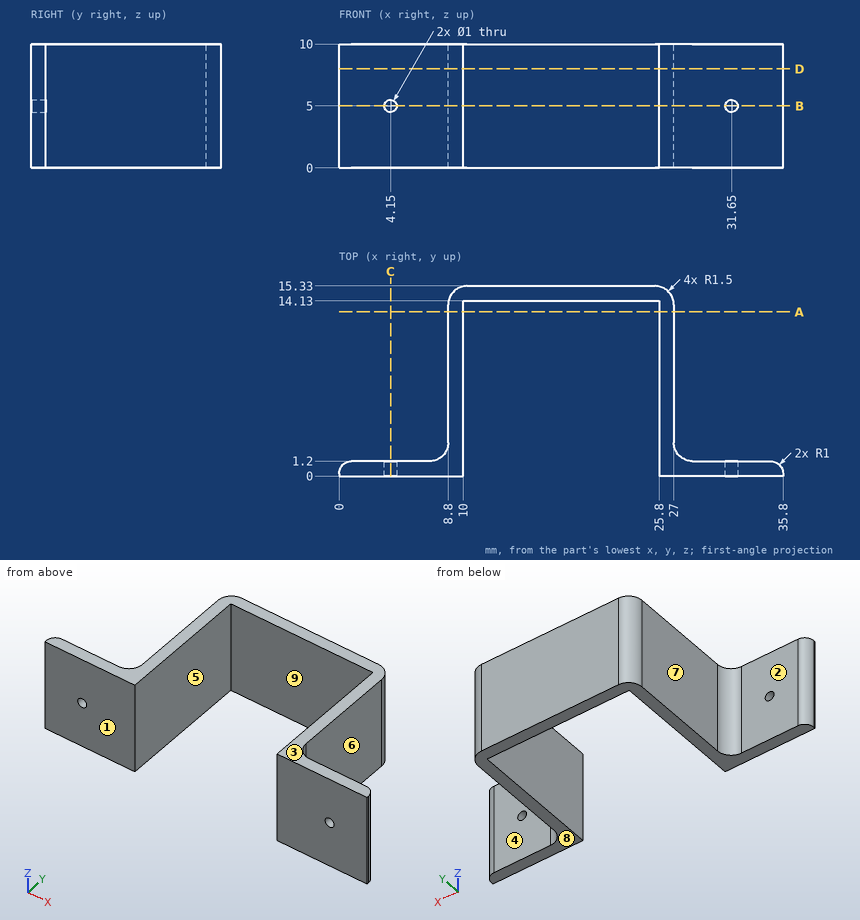
Geometry: see drawing. Coordinates: mm, zero at the bounding-box minimum. A direction names the side the tool comes from. Give positions to 0.01 mm unless a question says otherwise; leave off trailing zeros. Order: outer loops, then holes, each group sorted by start corner. A loop starts at its lowest first (then second) coordinate and runs counter-clockwise, first axis right, second up.
Q1. Section A-A on y = 13.25. Output: boundary loops of the cut face in (x, z), and give its area (3 significant figures).
Checked values:
outline: (8.8, 0) - (10, 0) - (10, 10) - (8.8, 10) - close; (25.8, 0) - (27, 0) - (27, 10) - (25.8, 10) - close
area: 24.0 mm2
Q2. Section C-C on x = 4.15. Output: boundary loops of the cut face in (y, z).
Checked values:
outline: (0, 0) - (1.2, 0) - (1.2, 4.5) - (0, 4.5) - close; (0, 5.5) - (1.2, 5.5) - (1.2, 10) - (0, 10) - close
Q3. Section D-D on z = 8. Output: boundary loops of the cut face in (x, y), and give its area (3 significant figures).
Checked values:
outline: (0, 0) - (10, 0) - (10, 14.13) - (25.8, 14.13) - (25.8, 0) - (35.8, 0) - (35.8, 0.2) arc R1 ccw to (34.8, 1.2) - (28.5, 1.2) arc R1.5 cw to (27, 2.7) - (27, 13.83) arc R1.5 ccw to (25.5, 15.33) - (10.3, 15.33) arc R1.5 ccw to (8.8, 13.83) - (8.8, 2.7) arc R1.5 cw to (7.3, 1.2) - (1, 1.2) arc R1 ccw to (0, 0.2) - close
area: 76.4 mm2
Q4. Draft query along X for the marked faces 6, 7, 8 and 9. Return one class per face: +X half, -X half, draft (parallel to the pull), parting line (faces both ways), or undercut.
Checked values:
face 6: +X half
face 7: -X half
face 8: draft
face 9: undercut
Q5. Ray query, probe 1 along X at (y, z) = (0.9, 5); probe 2 along X at (y, z) = (0.8, 5); probe 3 along X at (y, z) = (6, 5). Return the intervals inside material, ascending.
Checked values:
probe 1: x = 0.29 to 3.65, 4.65 to 10, 25.8 to 31.15, 32.15 to 35.51
probe 2: x = 0.2 to 3.65, 4.65 to 10, 25.8 to 31.15, 32.15 to 35.6
probe 3: x = 8.8 to 10, 25.8 to 27
Q6. Contact query for flat-ended pins moving along their axis: pin 1 Ø2 at (y, z) = (11, 3.5) entering from -X; pin 2 Ø5 at (y, z) = (7.5, 7.5) entering from +X; pin 3 Ø5 at (x, z) = (4, 6.5) entering from +Y; pin 4 Ø5 at (x, y) = (12, 8) entering from +Z. Output: stop coordinate, or through.
Checked values:
pin 1: stops at x = 8.8
pin 2: stops at x = 27
pin 3: stops at y = 1.2
pin 4: stops at z = 10
Q7. Section B-B on z = 5. Output: boundary loops of the cut face in (x, y).
Checked values:
outline: (0, 0) - (3.65, 0) - (3.65, 1.2) - (1, 1.2) arc R1 ccw to (0, 0.2) - close; (4.65, 0) - (10, 0) - (10, 14.13) - (25.8, 14.13) - (25.8, 0) - (31.15, 0) - (31.15, 1.2) - (28.5, 1.2) arc R1.5 cw to (27, 2.7) - (27, 13.83) arc R1.5 ccw to (25.5, 15.33) - (10.3, 15.33) arc R1.5 ccw to (8.8, 13.83) - (8.8, 2.7) arc R1.5 cw to (7.3, 1.2) - (4.65, 1.2) - close; (32.15, 0) - (35.8, 0) - (35.8, 0.2) arc R1 ccw to (34.8, 1.2) - (32.15, 1.2) - close
Q8. Set-up query: the marked faces 1, 2, 3, 4 and 5. Return all of +Z, -Z, +X, -X, +Y, -Y with unobstructed straight access to the full face (end or side cutting, diameter ignored); none if empty.
Checked values:
face 1: +Z, -Z, +X, -X, -Y
face 2: +Z, -Z, -X, +Y
face 3: +Z, +X, -X, +Y, -Y
face 4: +Z, -Z, +X, +Y
face 5: +Z, -Z, -Y
